Check sheet for the modelled part. Datum: model origin and axes. Units: mm. Face numbers are marked on the shaded views. A direction names the side the tool comes from. Give positions to 0.01 mm unless a question says otherwise; leave off trailing zeros. Write each loop counter-clockwise with the first axis right and the second up, starting at its lowest first coordinate (ties: lowest second). Pieces come first, ordered by that corner, then holes. Notation, with made-up numbers: (32, 85.5) -> (75, 85.5) arc R17 cw to (75, 96.5) -> close; hole circle Ø6 at (14.25, 83). An arc over 180 degrees is marked (long way). Use a Markdown table: item, result. Add a question column.
1. Cross-section at A-A (y = 0). Enter the section's corners in (x, z).
2. Cross-section at B-B (z = 3.5). Enter the section's corners in (x, y).
3. Cross-section at C-C (x = -0.5). Enter the section's corners in (y, z).
4. Release check for a two-part mould opening along Y. For the marked faces 6, 7, 8 and 9 record: released by +Y, released by -Y, zero draft, split by the parting line, or undercut.
5. Cross-section at D-D (z = 1.5). Enter the section's corners in (x, y), then the cut area to 3 significant figures.
6. Set-up check for the marked faces 1, 2, 3, 4 and 5: record each of +Z, -Z, +X, -X, +Y, -Y from which the full face is reachable in a straight line by a thin tool's end or side.
7. Gauge pin test, flat end, axial feed: P1, Ø2, axis at x = 0, y = 1, coming from the -Z side. Record the tip position at first contact, or that the pin passes through.
8. Scan lines: probe 1 along Y at (x, z) = (0, 1.4); probe 2 along Y at (x, z) = (1.3, 5.5); probe 3 along Y at (x, z) = (-0.8, 1.75). Record each from-to range of solid material in increasing order. Write a range as [from, to].
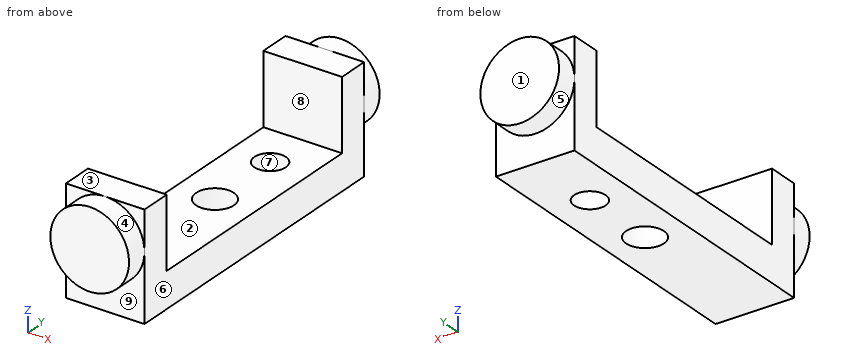
from build123d import *

# Parameters (mm, degrees)
SKETCH_1_W      = 5
SKETCH_1_H      = 19.865848542
SKETCH_1_R      = 1.200000017
SKETCH_1_R_2    = 1.000000001
EXTRUDE_1_DEPTH = 2.25
SKETCH_2_W      = 5
SKETCH_2_H      = 2
EXTRUDE_2_DEPTH = 4.5
SKETCH_3_R      = 2.5
EXTRUDE_3_DEPTH = 1.4


with BuildPart() as part:
    # Sketch 1 → Extrude 1 (new body)
    with BuildSketch(Plane.XY):
        Rectangle(SKETCH_1_W, SKETCH_1_H)
        with Locations((-3.5e-08, -2.5e-08)):
            Circle(SKETCH_1_R, mode=Mode.SUBTRACT)
        with Locations((1.04e-07, 4.982520103)):
            Circle(SKETCH_1_R_2, mode=Mode.SUBTRACT)
    extrude(amount=EXTRUDE_1_DEPTH)

    # Sketch 2 → Extrude 2 (add)
    with BuildSketch(Plane.XY.offset(2.25)):
        with Locations((0, 8.932924271)):
            Rectangle(SKETCH_2_W, SKETCH_2_H)
        with Locations((0, -8.932924271)):
            Rectangle(SKETCH_2_W, SKETCH_2_H)
    extrude(amount=EXTRUDE_2_DEPTH)

    # Sketch 3 → Extrude 3 (add)
    with BuildSketch(Plane(origin=(0, 9.932924271, 0), x_dir=(1, 0, 0), z_dir=(0, 1, 0))):
        with Locations(Location((0, -4.25, 0), (0, 0, 270))):
            Circle(SKETCH_3_R)
    extrude_3 = extrude(amount=EXTRUDE_3_DEPTH)

    # Mirror 1: Extrude 3 across plane
    add(extrude_3.mirror(Plane.ZX))


solid = part.part
Worked answers:
| question | item | result |
|---|---|---|
| 1 | outline | (-2.5, 0) -> (-1.2, 0) -> (-1.2, 2.25) -> (-2.5, 2.25) -> close; (1.2, 0) -> (2.5, 0) -> (2.5, 2.25) -> (1.2, 2.25) -> close |
| 2 | outline | (-2.5, -9.93) -> (-2.38, -9.93) -> (-2.38, -11.33) -> (2.38, -11.33) -> (2.38, -9.93) -> (2.5, -9.93) -> (2.5, -7.93) -> (-2.5, -7.93) -> close; (-2.5, 7.93) -> (2.5, 7.93) -> (2.5, 9.93) -> (2.38, 9.93) -> (2.38, 11.33) -> (-2.38, 11.33) -> (-2.38, 9.93) -> (-2.5, 9.93) -> close |
| 3 | outline | (-11.33, 1.8) -> (-9.93, 1.8) -> (-9.93, 0) -> (-1.09, 0) -> (-1.09, 2.25) -> (-7.93, 2.25) -> (-7.93, 6.75) -> (-9.93, 6.75) -> (-9.93, 6.7) -> (-11.33, 6.7) -> close; (1.09, 0) -> (4.12, 0) -> (4.12, 2.25) -> (1.09, 2.25) -> close; (5.85, 0) -> (9.93, 0) -> (9.93, 1.8) -> (11.33, 1.8) -> (11.33, 6.7) -> (9.93, 6.7) -> (9.93, 6.75) -> (7.93, 6.75) -> (7.93, 2.25) -> (5.85, 2.25) -> close |
| 4 | face 6 | zero draft |
| 4 | face 7 | undercut |
| 4 | face 8 | undercut |
| 4 | face 9 | released by -Y |
| 5 | outline | (-2.5, -9.93) -> (2.5, -9.93) -> (2.5, 9.93) -> (-2.5, 9.93) -> close; hole circle Ø2.4 at (0, 0); hole circle Ø2 at (0, 4.98) |
| 5 | area | 91.7 mm² |
| 6 | face 1 | +Z, -Z, +X, -X, +Y |
| 6 | face 2 | +Z, +X, -X |
| 6 | face 3 | +Z, +X, -X, +Y, -Y |
| 6 | face 4 | -Y |
| 6 | face 5 | +Y |
| 7 | P1 | stops at z = 0 |
| 8 | probe 1 | y = [-9.93, -1.2], [1.2, 3.98], [5.98, 9.93] |
| 8 | probe 2 | y = [-11.33, -7.93], [7.93, 11.33] |
| 8 | probe 3 | y = [-9.93, -0.89], [0.89, 4.38], [5.58, 9.93] |
